Study the drawing (mm; zero at the part's minimum x, y, z) and answer. Round coordinates to 2 decimals unless told otherwise and drop trailing zeros. Write each loop counter-clockwise with the first axis right and the second up, starting at its lowest first coordinate (ties: lowest second). Pieces come first, ordered by that corner, then holes.
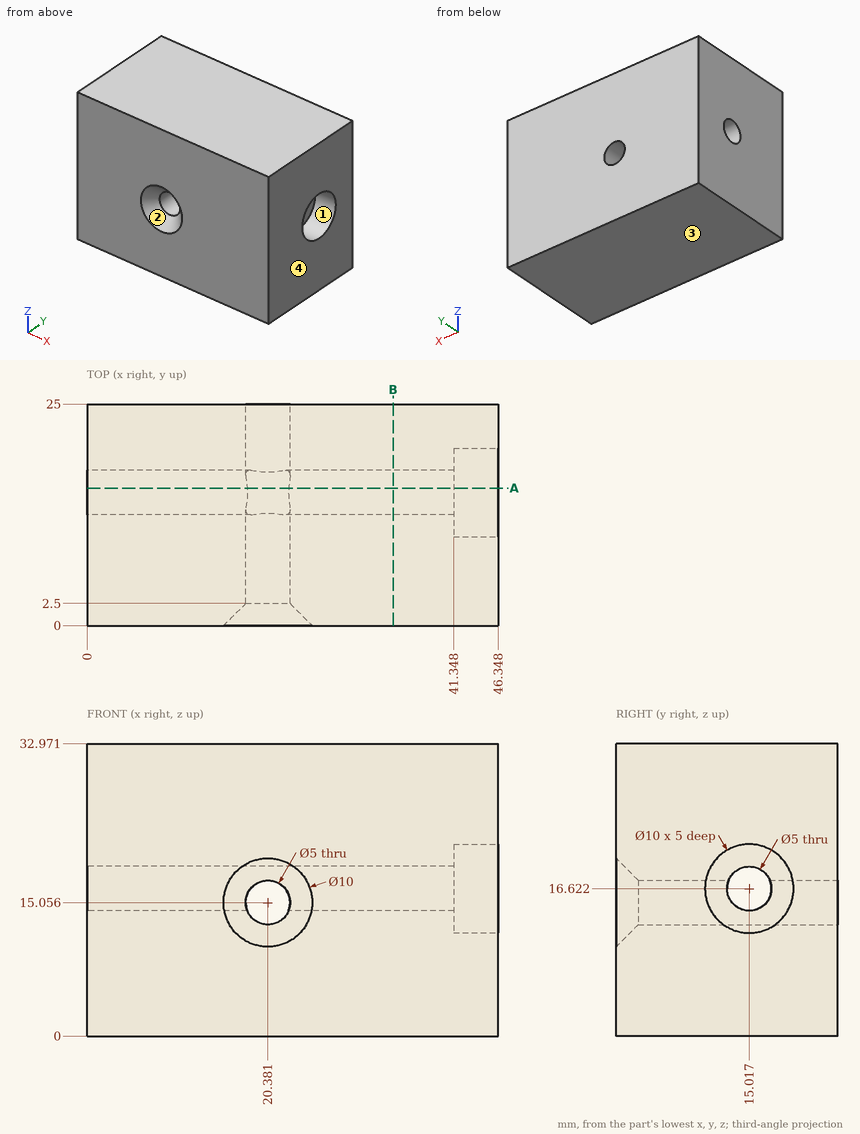
1. Section A-A on y = 15.5 is taken. Determine the outline of the cut face in (x, z) (1 decimal), plus the area to 3 significant figures.
Geometry says:
outline: (0, 0) - (46.3, 0) - (46.3, 11.6) - (41.3, 11.6) - (41.3, 14.2) - (22.7, 14.2) arc R2.5 cw to (18, 14.2) - (0, 14.2) - close; (0, 19.1) - (41.3, 19.1) - (41.3, 21.6) - (46.3, 21.6) - (46.3, 33) - (0, 33) - close
area: 1,270 mm2
2. Given pin 1 (6.5 mm diameter, centred on x = 20.38, z = 15.06, fed in from -Y) (1 decimal); pin 2 (5 mm diameter, centred on y = 13.5, z = 18, fed in from +X), each flat-ended and moving along its own axis, determine where each tip first touches the part or whether it passes through.
Geometry says:
pin 1: stops at y = 1.7
pin 2: stops at x = 41.35
3. Straight lines are drawn through the part: line 1 along Z through (x, y) = (21, 23.75) (1 decimal); line 2 along Z through (x, y) = (35.5, 16.25); line 3 along X through (y, z) = (18, 20). For each, find the intervals that lie inside material, in ascending order.
Geometry says:
line 1: z = 0 to 12.6, 17.5 to 33
line 2: z = 0 to 14.45, 18.8 to 32.97
line 3: x = 0 to 41.35
4. Section B-B on x = 34.5 is taken. Determine the outline of the cut face in (y, z).
Geometry says:
outline: (0, 0) - (25, 0) - (25, 32.97) - (0, 32.97) - close; hole circle Ø5 at (15.02, 16.62)
5. For a pull along Z with two mould halves and no side action, classify the marked faces 1, 2, 3 and 4 as released by +Z, released by -Z, zero draft, split by the parting line, or undercut.
Geometry says:
face 1: undercut
face 2: undercut
face 3: released by -Z
face 4: zero draft
